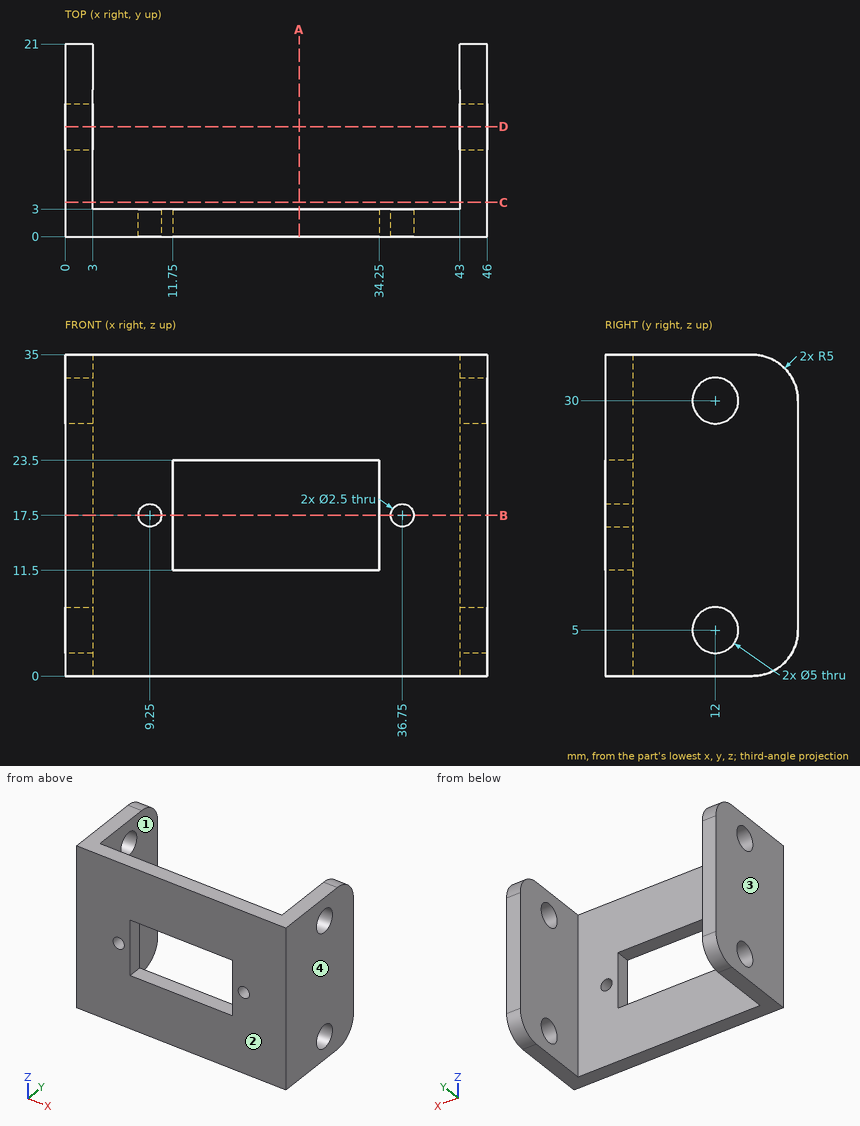
Can you work these out from the drawing? Everything is in mm from the part's minimum corner. Give positions to 0.01 mm unless a question says otherwise; leave off trailing zeros. Write each loop counter-clockwise with the first axis right and the second up, starting at its lowest first coordinate (ties: lowest second). Pieces come first, ordered by that corner, then holes. Notation, with made-up numbers: (20, 5.25) -> (39, 5.25) arc R11 cw to (39, 16.25) -> close; hole circle Ø7 at (86.25, 39.25). An arc over 180 degrees is marked (long way). Write each question's results on one line, items separated by ' | '.
Item 1: Suppose I cut it at C-C on y = 3.75. Write out the boundary of the cut face in (x, z), plus the area to 3 significant figures.
Output:
outline: (0, 0) -> (3, 0) -> (3, 35) -> (0, 35) -> close; (43, 0) -> (46, 0) -> (46, 35) -> (43, 35) -> close | area: 210 mm^2
Item 2: Suppose I cut it at B-B on z = 17.5. Write out the boundary of the cut face in (x, y), plus the area to 4 significant figures.
Output:
outline: (0, 0) -> (8, 0) -> (8, 3) -> (3, 3) -> (3, 21) -> (0, 21) -> close; (10.5, 0) -> (11.75, 0) -> (11.75, 3) -> (10.5, 3) -> close; (34.25, 0) -> (35.5, 0) -> (35.5, 3) -> (34.25, 3) -> close; (38, 0) -> (46, 0) -> (46, 21) -> (43, 21) -> (43, 3) -> (38, 3) -> close | area: 163.5 mm^2
Item 3: We'd pull the mould along X, two halves only. Please class the marked faces 1, 2, 3 and 4: pulls with the +X half, pulls with the -X half, needs draft (parallel to the pull), parting line crosses it, or undercut.
Output:
face 1: undercut | face 2: needs draft | face 3: pulls with the -X half | face 4: pulls with the +X half
Item 4: If I drill on L1, parallel to X at y = 15.25, z = 2; L2, parallel to Y at x = 43.6, z = 30; L3, parallel to Z at x = 18.5, y = 1.5, over which ranges is the centre line in solid material (lowest first)?
Output:
L1: x = 0 to 3, 43 to 46 | L2: y = 0 to 9.5, 14.5 to 21 | L3: z = 0 to 11.5, 23.5 to 35
Item 5: Suppose I cut it at D-D on y = 12. Write out the boundary of the cut face in (x, z), plus the area to 3 significant figures.
Output:
outline: (0, 0) -> (3, 0) -> (3, 2.5) -> (0, 2.5) -> close; (0, 7.5) -> (3, 7.5) -> (3, 27.5) -> (0, 27.5) -> close; (0, 32.5) -> (3, 32.5) -> (3, 35) -> (0, 35) -> close; (43, 0) -> (46, 0) -> (46, 2.5) -> (43, 2.5) -> close; (43, 7.5) -> (46, 7.5) -> (46, 27.5) -> (43, 27.5) -> close; (43, 32.5) -> (46, 32.5) -> (46, 35) -> (43, 35) -> close | area: 150 mm^2
Item 6: For pin 1 Ø1.5 at (x, z) = (29, 6) entering from -Y, with a flat end and sliding along its axis, tell me the tip position at first contact or that it passes through.
Output:
pin 1: stops at y = 0
Item 7: Suppose I cut it at A-A on x = 25.5. Write out the boundary of the cut face in (y, z), plus the area to 3 significant figures.
Output:
outline: (0, 0) -> (3, 0) -> (3, 11.5) -> (0, 11.5) -> close; (0, 23.5) -> (3, 23.5) -> (3, 35) -> (0, 35) -> close | area: 69.0 mm^2
